Source: CAD feature listing. Evaluate the final solid. Frame: model axes, mm. Face numbers are marked on the shaded views. Give positions to 0.01 mm unless a question says otherwise; leave off trailing zeros. Loops run counter-clockwise (first coordinate to the right, second up) from the corner with the lowest first, then second, coordinate; pieces in that order, holes last.
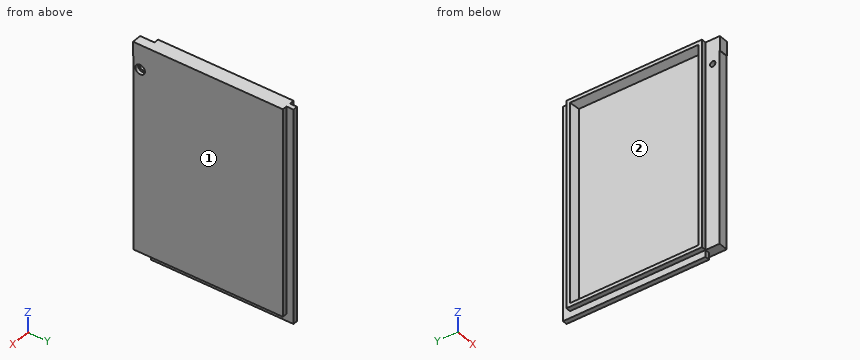
from build123d import *
from OCP.BRepFilletAPI import BRepFilletAPI_MakeChamfer

# Parameters (mm, degrees)
SKETCH2_W           = 95
SKETCH2_H           = 145
BOSS_EXTRUDE1_DEPTH = 10
SKETCH3_W           = 3.3
SKETCH3_H           = 4.8
BOSS_EXTRUDE3_DEPTH = 95
SKETCH4_W           = 3.3
SKETCH4_H           = 149.8
BOSS_EXTRUDE4_DEPTH = 4.9
BOSS_EXTRUDE5_DEPTH = 10
CUT_EXTRUDE1_REACH  = 178.366
SKETCH6_R           = 1.9
SKETCH8_R           = 3.35
CUT_EXTRUDE3_DEPTH  = 2.5
CUT_EXTRUDE2_REACH  = 178.366
SKETCH7_W           = 0.2
SKETCH7_H           = 135
SKETCH9_W           = 85
SKETCH9_H           = 135
CUT_EXTRUDE4_DEPTH  = 5
CHAMFER1_SIZE       = 2.5
CHAMFER1_SIZE_2     = 5


with BuildPart() as part:
    # Sketch2 → Boss-Extrude1 (new body)
    with BuildSketch(Plane.YZ):
        with Locations((47.5, 72.5)):
            Rectangle(SKETCH2_W, SKETCH2_H)
    extrude(amount=BOSS_EXTRUDE1_DEPTH)

    # Sketch3 → Boss-Extrude3 (add)
    with BuildSketch(Plane(origin=(0, 95, 0), x_dir=(-1, 0, 0), z_dir=(0, 1, 0))):
        with Locations((-5, -2.4)):
            Rectangle(SKETCH3_W, SKETCH3_H)
    extrude(amount=-BOSS_EXTRUDE3_DEPTH)

    # Sketch4 → Boss-Extrude4 (add)
    with BuildSketch(Plane(origin=(0, 95, 0), x_dir=(-1, 0, 0), z_dir=(0, 1, 0))):
        with Locations((-5, 70.1)):
            Rectangle(SKETCH4_W, SKETCH4_H)
    extrude(amount=BOSS_EXTRUDE4_DEPTH)

    # Sketch5 → Boss-Extrude5 (add)
    with BuildSketch(Plane.XZ):
        Polygon((10, 145), (3.35, 145), (3.35, 0), (6.65, 0), (10, 0), align=None)
    extrude(amount=BOSS_EXTRUDE5_DEPTH)

    # Sketch6 → Cut-Extrude1 (cut, up to next)
    with BuildSketch(Plane.YZ.offset(10), mode=Mode.PRIVATE) as cut_extrude1_sk1:
        with Locations(Location((-5, 127.75, 0), (0, 0, 270))):
            Circle(SKETCH6_R)
    cut_extrude1_tool1 = extrude(cut_extrude1_sk1.sketch, amount=-CUT_EXTRUDE1_REACH, mode=Mode.PRIVATE) & part.part
    add(cut_extrude1_tool1.solids().sort_by_distance((10, -5, 127.75))[0], mode=Mode.SUBTRACT)

    # Sketch8 → Cut-Extrude3 (cut)
    with BuildSketch(Plane.YZ.offset(10)):
        with Locations(Location((-5, 127.75, 0), (0, 0, 270))):
            Circle(SKETCH8_R)
    extrude(amount=-CUT_EXTRUDE3_DEPTH, mode=Mode.SUBTRACT)

    # Sketch7 → Cut-Extrude2 (cut, up to next)
    with BuildSketch(Plane.YZ.offset(10), mode=Mode.PRIVATE) as cut_extrude2_sk1:
        with Locations((-9.9, 67.5)):
            Rectangle(SKETCH7_W, SKETCH7_H)
    cut_extrude2_tool1 = extrude(cut_extrude2_sk1.sketch, amount=-CUT_EXTRUDE2_REACH, mode=Mode.PRIVATE) & part.part
    add(cut_extrude2_tool1.solids().sort_by_distance((10, -9.9, 67.5))[0], mode=Mode.SUBTRACT)

    # Sketch9 → Cut-Extrude4 (cut)
    with BuildSketch(Plane(origin=(0, 0, 0), x_dir=(0, -1, 0), z_dir=(-1, 0, 0))):
        with Locations((-47.5, 72.5)):
            Rectangle(SKETCH9_W, SKETCH9_H)
    extrude(amount=-CUT_EXTRUDE4_DEPTH, mode=Mode.SUBTRACT)

    # Chamfer1
    chamfer1_edges_1 = [part.edges().sort_by_distance(p)[0] for p in [
        (0, 47.5, 5),
    ]]
    chamfer1_side_1 = [part.faces().sort_by_distance(p)[0] for p in [
        (0, 47.5, 4.95),
    ]]
    chamfer1_edges_2 = [part.edges().sort_by_distance(p)[0] for p in [
        (0, 5, 72.5),
    ]]
    chamfer1_side_2 = [part.faces().sort_by_distance(p)[0] for p in [
        (0, 4.95, 72.5),
    ]]
    chamfer1_edges_3 = [part.edges().sort_by_distance(p)[0] for p in [
        (0, 90, 72.5),
    ]]
    chamfer1_side_3 = [part.faces().sort_by_distance(p)[0] for p in [
        (0, 90.05, 72.5),
    ]]
    chamfer1_edges_4 = [part.edges().sort_by_distance(p)[0] for p in [
        (0, 47.5, 140),
    ]]
    chamfer1_side_4 = [part.faces().sort_by_distance(p)[0] for p in [
        (0, 47.5, 140.05),
    ]]
    chamfer1 = BRepFilletAPI_MakeChamfer(part.part.solid().wrapped)
    for e in chamfer1_edges_1:
        chamfer1.Add(CHAMFER1_SIZE - 0.0001, CHAMFER1_SIZE_2 - 0.0001, e.wrapped, chamfer1_side_1[0].wrapped)
    for e in chamfer1_edges_2:
        chamfer1.Add(CHAMFER1_SIZE - 0.0001, CHAMFER1_SIZE_2 - 0.0001, e.wrapped, chamfer1_side_2[0].wrapped)
    for e in chamfer1_edges_3:
        chamfer1.Add(CHAMFER1_SIZE - 0.0001, CHAMFER1_SIZE_2 - 0.0001, e.wrapped, chamfer1_side_3[0].wrapped)
    for e in chamfer1_edges_4:
        chamfer1.Add(CHAMFER1_SIZE - 0.0001, CHAMFER1_SIZE_2 - 0.0001, e.wrapped, chamfer1_side_4[0].wrapped)
    add(Compound.cast(chamfer1.Shape()), mode=Mode.REPLACE)  # a hair under: the kernel refuses the full size


solid = part.part
1) Ray query, probe 1 along Y at (x, z) = (5.85, 127.75); probe 2 along Y at (x, z) = (9.2, 127.75); probe 3 along Z at (x, y) = (9.75, 93). Return the intervals inside material, ascending.
Checks:
probe 1: y = -9.8 to -6.9, -3.1 to 99.9
probe 2: y = -9.8 to -8.35, -1.65 to 95
probe 3: z = 0 to 145
2) Cut plane A-A (y = -5). Return loops of the section in (x, z), and give its area (3 significant figures).
Checks:
outline: (3.35, 0) - (10, 0) - (10, 124.4) - (7.5, 124.4) - (7.5, 125.85) - (3.35, 125.85) - close; (3.35, 129.65) - (7.5, 129.65) - (7.5, 131.1) - (10, 131.1) - (10, 145) - (3.35, 145) - close
area: 932 mm2
3) Pull-direction query (Z, two-part tool) for the marked faces 1 and 2; classes: released by +Z, released by -Z, zero draft, split by the parting line, or undercut.
Checks:
face 1: zero draft
face 2: undercut
4) Contact query for flat-ended pins moving along their axis: P1, Ø8, axis at y = -6.5, z = 68, coming from the -X side; P2, Ø4, axis at y = 26.5, z = 15.5, coming from the -X side; P3, Ø1.7, axis at x = 2, z = 71.5, coming from the -Y side. Output: stop coordinate, or through.
Checks:
P1: stops at x = 3.35
P2: stops at x = 5
P3: stops at y = 0
